Can you work these out from the model? Positions are in its coordinate system, mm. A direction names the side the tool comes from. Round coordinates to 2 decimals unless told otherwise and drop trailing zeros. Loops run counter-clockwise (first coordinate to the right, second up) from the corner with the lowest first, then second, coordinate; pieces in that order, holes last.
(1) I want a section at C-C on x = 1.5. Write out the boundary of the cut face in (y, z).
(2) Thinking about a two-plate mould opening in Y: for faces 3 (the face through (13, 0, 6.35)), 4 (the face through (-6.35, -0.14, 0.09)), 5 (the face through (21.5, 1, 0.1)), 6 (the face through (1.89, -1.45, -0.09)), which applies, released by +Y, released by -Y, zero draft, split by the parting line, or undercut?
(3) I want a section at A-A on y = 0. Write out the boundary of the cut face in (x, z), plus the area to 3 significant figures.
(4) Will these pins go through, and if not, where does the flat tip stop? pin 1 Ø5 at (y, z) = (-5, 3) entering from -X; pin 2 Ø4 at (x, z) = (-2.5, -0.5) entering from +Y; pin 3 Ø6 at (y, z) = (4.5, -4) entering from -X.
(5) Which directions (+Z, -Z, +X, -X, +Y, -Y) give clear straight access to the entire face, cutting with the end or side of a thin tool? Please do faces 1 (the face through (13, 0, -6.35)), 2 (the face through (20.9, 0, 0)).
(6) I want a section at B-B on z = 2. Write out the boundary of the cut face in (x, y), plus the area to 3 significant figures.
(7) I want a section at D-D on y = 3. Write out the boundary of the cut face in (x, z).
(8) If I drill on line 1 along Y through (x, z) = (0, 2.25); line 2 along Y through (x, z) = (25.4, -0.75); line 3 along X through (y, z) = (-0.5, -3), over which ranges is the centre line in solid material (lowest first)?
from build123d import *

# Parameters (mm, degrees)
MAIN_BODY_DEPTH                = 6.35
F_3_16_0_1875_DIAMETER_HOLE1_D = 4.7625
F_7_0_7_DIAMETER_HOLE1_D       = 7
F_7_0_7_DIAMETER_HOLE1_DEPTH   = 12.7
F_7_0_7_DIAMETER_HOLE1_TIP     = 2.103012167
SKETCH6_W                      = 2.5
SKETCH6_H                      = 2
CUT_2X2_KEYWAY_DEPTH           = 35.780382402


with BuildPart() as part:
    # Sketch1 → Main Body (new, symmetric)
    with BuildSketch(Plane.XY):
        with BuildLine():
            Line((0, 6.35), (25.4, 6.35))
            ThreePointArc((25.4, 6.35), (31.75, 0), (25.4, -6.35))
            Line((25.4, -6.35), (0, -6.35))
            ThreePointArc((0, -6.35), (-6.35, 0), (0, 6.35))
        make_face()
    extrude(amount=MAIN_BODY_DEPTH, both=True)

    # 3/16 (0.1875) Diameter Hole1 (through all)
    with Locations(Plane.XY.offset(6.35)):
        with Locations((0, 0)):
            Hole(F_3_16_0_1875_DIAMETER_HOLE1_D / 2)

    # Ø7.0 (7) Diameter Hole1
    with Locations(Plane.XY.offset(6.35)):
        with Locations((25.4, 0)):
            Hole(F_7_0_7_DIAMETER_HOLE1_D / 2, depth=F_7_0_7_DIAMETER_HOLE1_DEPTH)
            with Locations((0, 0, -(F_7_0_7_DIAMETER_HOLE1_DEPTH + F_7_0_7_DIAMETER_HOLE1_TIP / 2))):  # 118° drill point
                Cone(0, F_7_0_7_DIAMETER_HOLE1_D / 2, F_7_0_7_DIAMETER_HOLE1_TIP, mode=Mode.SUBTRACT)

    # Sketch6 → Cut-2x2 Keyway (cut, through all)
    with BuildSketch(Plane.XY.offset(6.35)):
        with Locations((22.15, 0)):
            Rectangle(SKETCH6_W, SKETCH6_H)
    extrude(amount=-CUT_2X2_KEYWAY_DEPTH, mode=Mode.SUBTRACT)


solid = part.part
Filled sheet:
1. outline: (-6.35, -6.35) - (-1.85, -6.35) - (-1.85, 6.35) - (-6.35, 6.35) - close; (1.85, -6.35) - (6.35, -6.35) - (6.35, 6.35) - (1.85, 6.35) - close
2. face 3: zero draft
2. face 4: split by the parting line
2. face 5: undercut
2. face 6: undercut
3. outline: (-6.35, -6.35) - (-2.38, -6.35) - (-2.38, 6.35) - (-6.35, 6.35) - close; (2.38, -6.35) - (20.9, -6.35) - (20.9, 6.35) - (2.38, 6.35) - close; (28.9, -6.35) - (31.75, -6.35) - (31.75, 6.35) - (28.9, 6.35) - close
3. area: 322 mm2
4. pin 1: stops at x = -5.84
4. pin 2: stops at y = 6.33
4. pin 3: stops at x = -6.17
5. face 1: -Z, +X, -X, +Y, -Y
5. face 2: +Z, -Z
6. outline: (0, -6.35) - (25.4, -6.35) arc R6.35 ccw to (25.4, 6.35) - (0, 6.35) arc R6.35 ccw to start; hole circle Ø4.76 at (0, 0); hole (20.9, -1) - (22.05, -1) arc R3.5 ccw (long way) to (22.05, 1) - (20.9, 1) - close
6. area: 391 mm2
7. outline: (-5.6, -6.35) - (23.6, -6.35) - (23.6, 6.35) - (-5.6, 6.35) - close; (27.2, -6.35) - (31, -6.35) - (31, 6.35) - (27.2, 6.35) - close
8. line 1: y = -6.35 to -2.38, 2.38 to 6.35
8. line 2: y = -6.35 to -3.5, 3.5 to 6.35
8. line 3: x = -6.33 to -2.33, 2.33 to 20.9, 28.86 to 31.73
